from build123d import *

# Parameters (mm, degrees)
BOSS_EXTRUDE1_DEPTH = 2.5
CUT_EXTRUDE1_DEPTH  = 2.5
SKETCH3_R           = 1.75
CUT_EXTRUDE2_DEPTH  = 2.5
FILLET1_R           = 2


with BuildPart() as part:
    # Sketch1 → Boss-Extrude1 (new body)
    with BuildSketch(Plane.XY):
        with BuildLine():
            Line((-5, 6.244997998), (-5, 7.5))
            Line((-5, 7.5), (-10.998080575, 1.501919425))
            Line((-10.998080575, 1.501919425), (-11.001951051, -1.498048949))
            Line((-11.001951051, -1.498048949), (-5, -7.5))
            Line((-5, -7.5), (-5, -6.244997998))
            ThreePointArc((-5, -6.244997998), (-6.854583671, -4.124885779), (-7.859375, -1.493393655))
            ThreePointArc((-7.859375, -1.493393655), (-9.5, 0), (-7.859375, 1.493393655))
            ThreePointArc((-7.859375, 1.493393655), (-6.854583671, 4.124885779), (-5, 6.244997998))
        make_face()
        with BuildLine():
            Line((0, 9.499997384), (0, 11.00001831))
            Line((0, 11.00001831), (-1.498048949, 11.001951051))
            Line((-1.498048949, 11.001951051), (-5, 7.5))
            Line((-5, 7.5), (-5, 6.244997998))
            ThreePointArc((-5, 6.244997998), (-3.346805661, 7.266284599), (-1.496145717, 7.85885157))
            ThreePointArc((-1.496145717, 7.85885157), (-1.111300148, 9.010559559), (0, 9.499997384))
        make_face()
        with BuildLine():
            Line((1.501919425, 10.998080575), (0, 11.00001831))
            Line((0, 11.00001831), (0, 9.499997384))
            ThreePointArc((0, 9.499997384), (1.058848726, 9.059669249), (1.497198557, 8))
            ThreePointArc((1.497198557, 8), (1.495558351, 7.929872059), (1.490641319, 7.859897484))
            ThreePointArc((1.490641319, 7.859897484), (3.344260945, 7.267456139), (5, 6.244997998))
            Line((5, 6.244997998), (5, 7.5))
            Line((5, 7.5), (1.501919425, 10.998080575))
        make_face()
        with BuildLine():
            Line((11.001951051, 1.498048949), (5, 7.5))
            Line((5, 7.5), (5, 6.244997998))
            ThreePointArc((5, 6.244997998), (6.853793729, 4.126198193), (7.858802525, 1.496403311))
            ThreePointArc((7.858802525, 1.496403311), (9.007744437, 1.111312618), (9.497198557, 0.002801443))
            ThreePointArc((9.497198557, 0.002801443), (9.00813269, -1.105355666), (7.859848986, -1.490897019))
            ThreePointArc((7.859848986, -1.490897019), (6.855238728, -4.123797035), (5, -6.244997998))
            Line((5, -6.244997998), (5, -7.5))
            Line((5, -7.5), (10.998080575, -1.501919425))
            Line((10.998080575, -1.501919425), (11.001951051, 1.498048949))
        make_face()
        with BuildLine():
            ThreePointArc((-1.493650301, -7.859326229), (-3.345652024, -7.266815846), (-5, -6.244997998))
            Line((-5, -6.244997998), (-5, -7.5))
            Line((-5, -7.5), (-1.501919425, -10.998080575))
            Line((-1.501919425, -10.998080575), (0, -11.00001831))
            Line((0, -11.00001831), (0, -9.497198557))
            ThreePointArc((0, -9.497198557), (-1.108333995, -9.007938758), (-1.493650301, -7.859326229))
        make_face()
        with BuildLine():
            Line((5, -7.5), (5, -6.244997998))
            ThreePointArc((5, -6.244997998), (3.345652024, -7.266815846), (1.493650301, -7.859326229))
            ThreePointArc((1.493650301, -7.859326229), (1.498411734, -7.928189323), (1.5, -7.997198557))
            ThreePointArc((1.5, -7.997198557), (1.060660172, -9.057858728), (0, -9.497198557))
            Line((0, -9.497198557), (0, -11.00001831))
            Line((0, -11.00001831), (1.498048949, -11.001951051))
            Line((1.498048949, -11.001951051), (5, -7.5))
        make_face()
        with BuildLine():
            ThreePointArc((0, 6.500002616), (-1.011288975, 6.889615878), (-1.496145717, 7.85885157))
            ThreePointArc((-1.496145717, 7.85885157), (-3.346805661, 7.266284599), (-5, 6.244997998))
            Line((-5, 6.244997998), (-5, -6.244997998))
            ThreePointArc((-5, -6.244997998), (-3.345652024, -7.266815846), (-1.493650301, -7.859326229))
            ThreePointArc((-1.493650301, -7.859326229), (-1.010740201, -6.888864561), (0, -6.497198557))
            Line((0, -6.497198557), (0, 6.500002616))
        make_face()
        with BuildLine():
            Line((-5, -6.244997998), (-5, 6.244997998))
            ThreePointArc((-5, 6.244997998), (-6.854583671, 4.124885779), (-7.859375, 1.493393655))
            ThreePointArc((-7.859375, 1.493393655), (-6.890735041, 1.009718401), (-6.5, 0))
            ThreePointArc((-6.5, 0), (-6.890735041, -1.009718401), (-7.859375, -1.493393655))
            ThreePointArc((-7.859375, -1.493393655), (-6.854583671, -4.124885779), (-5, -6.244997998))
        make_face()
        with BuildLine():
            Line((5, -6.244997998), (5, 6.244997998))
            ThreePointArc((5, 6.244997998), (3.344260945, 7.267456139), (1.490641319, 7.859897484))
            ThreePointArc((1.490641319, 7.859897484), (1.008146228, 6.891855241), (0, 6.500002616))
            Line((0, 6.500002616), (0, -6.497198557))
            ThreePointArc((0, -6.497198557), (1.010740201, -6.888864561), (1.493650301, -7.859326229))
            ThreePointArc((1.493650301, -7.859326229), (3.345652024, -7.266815846), (5, -6.244997998))
        make_face()
        with BuildLine():
            ThreePointArc((7.858802525, 1.496403311), (6.853793729, 4.126198193), (5, 6.244997998))
            Line((5, 6.244997998), (5, -6.244997998))
            ThreePointArc((5, -6.244997998), (6.855238728, -4.123797035), (7.859848986, -1.490897019))
            ThreePointArc((7.859848986, -1.490897019), (6.497198649, 0.002275989), (7.858802525, 1.496403311))
        make_face()
    extrude(amount=BOSS_EXTRUDE1_DEPTH)

    # Sketch2 → Cut-Extrude1 (cut)
    with BuildSketch(Plane.XY.offset(2.5)):
        Polygon((-5, 5), (-10.998080575, 1.501919425), (-1.498048949, 11.001951051), align=None)
        Polygon((-5, -5), (-1.501919425, -10.998080575), (-11.001951051, -1.498048949), align=None)
        Polygon((1.501919425, 10.998080575), (5, 5), (11.001951051, 1.498048949), align=None)
        Polygon((10.998080575, -1.501919425), (5, -5), (1.498048949, -11.001951051), align=None)
    extrude(amount=-CUT_EXTRUDE1_DEPTH, mode=Mode.SUBTRACT)

    # Sketch3 → Cut-Extrude2 (cut)
    with BuildSketch(Plane.XY.offset(2.5)):
        Circle(SKETCH3_R)
    extrude(amount=-CUT_EXTRUDE2_DEPTH, mode=Mode.SUBTRACT)

    # Fillet1
    fillet1_edges = [part.edges().sort_by_distance(p)[0] for p in [
        (1.498048949, -11.001951051, 1.25),
        (-1.501919425, -10.998080575, 1.25),
        (-11.001951051, -1.498048949, 1.25),
        (-10.998080575, 1.501919425, 1.25),
        (-1.498048949, 11.001951051, 1.25),
        (1.501919425, 10.998080575, 1.25),
        (11.001951051, 1.498048949, 1.25),
        (10.998080575, -1.501919425, 1.25),
        (-5, -5, 1.25),
        (5, 5, 1.25),
        (5, -5, 1.25),
        (-5, 5, 1.25),
    ]]
    fillet(fillet1_edges, radius=FILLET1_R)


solid = part.part
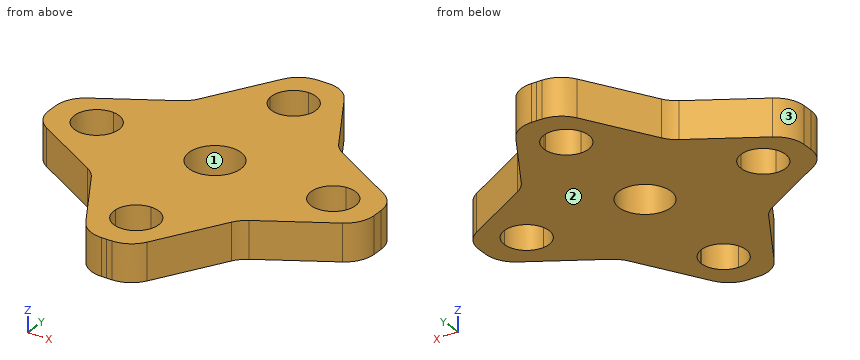
Geometry: final body of the model. Coordinates: model frame, mm. Face numbers are marked on the shaded views. Give positions to 0.01 mm unless a question says otherwise; leave off trailing zeros. Loops run counter-clockwise (first coordinate to the right, second up) from the corner with the lowest first, then second, coordinate; pieces in that order, holes last. Notation, with made-up numbers: (73, 31.5) - (78, 31.5) arc R37 ccw to (78, 68.5) - close; hole circle Ø4 at (-33.75, 10). An arc over 180 degrees is marked (long way). Answer as CSV lines item,"result". Start each with the question number.
1. Section B-B, the plane z = 1.5. Give the number of separate pieces and of enclosed holes in the cut face, plus the area to 3 significant figures.
2. Section C-C, the plane x = 9.75. Return loops of the section in (y, z).
3. Section D-D, the plane x = -6.25. Return loops of the section in (y, z), plus the area to 3 significant figures.
4. Ray query, L1, parallel to X at y = 0.25, z = 2.25; L2, parallel to Y at x = -1, z = 0.2. Return the intervals inside material, ascending.
5. Pin query (flat end, axial travel): P1, Ø1.5, axis at y = -5.5, z = 1.5, coming from the -X side. Return the tip coordinate at first contact, or that it passes through.
6. Section A-A, the plane x = 0.75. Return loops of the section in (y, z).
7. Draft query along Y for the marked faces 1, 2 and 3. Return one class per face: released by +Y, released by -Y, zero draft, split by the parting line, or undercut.
Answers:
1,separate pieces,"1"
1,enclosed holes,"5"
1,area,"217 mm2"
2,outline,"(-2.23, 0) - (2.23, 0) - (2.23, 2.5) - (-2.23, 2.5) - close"
3,outline,"(-4.27, 0) - (4.27, 0) - (4.27, 2.5) - (-4.27, 2.5) - close"
3,area,"21.4 mm2"
4,L1,"x = -11 to -9.48, -6.52 to -1.73, 1.73 to 6.52, 9.48 to 11"
4,L2,"y = -10.89 to -9.12, -6.88 to -1.44, 1.44 to 6.88, 9.12 to 10.89"
5,P1,"stops at x = -5.43"
6,outline,"(-10.96, 0) - (-9.3, 0) - (-9.3, 2.5) - (-10.96, 2.5) - close; (-6.7, 0) - (-1.58, 0) - (-1.58, 2.5) - (-6.7, 2.5) - close; (1.58, 0) - (6.7, 0) - (6.7, 2.5) - (1.58, 2.5) - close; (9.3, 0) - (10.96, 0) - (10.96, 2.5) - (9.3, 2.5) - close"
7,face 1,"undercut"
7,face 2,"zero draft"
7,face 3,"released by +Y"
